```python
from build123d import *

# Parameters (mm, degrees)
F0_R           = 136.525
F1_DEPTH       = 3.175
F3_D           = 4.9784
F3_CSINK_D     = 9.8298
F3_CSINK_ANGLE = 82


with BuildPart() as f1:
    # F0 (on Top) → F1 (new body)
    with BuildSketch(Plane.XY):
        Circle(F0_R)
    extrude(amount=-F1_DEPTH)

    # F3 (through all)
    with Locations(Plane.XY):
        with Locations((-114.3, 0), (-57.15, 98.986704), (57.15, 98.986704), (114.3, 0), (57.15, -98.986704), (-57.15, -98.986704)):
            CounterSinkHole(F3_D / 2, F3_CSINK_D / 2, counter_sink_angle=F3_CSINK_ANGLE)


solid = f1.part
```
Read the model definition and answer for the solid it produces. Units are mm, in the model's axes. Coordinates: 2 decimals unless noted, no trailing zeros. Order: outer loops, then holes, each group sorted by start corner. A loop starts at its lowest first (then second) coordinate and runs counter-clockwise, first axis right, second up. Notation, with made-up numbers: (34, -17) - (75, -17) arc R20 ccw to (75, -11) - close; hole circle Ø3 at (15, 3.25). An arc over 180 degrees is marked (long way). Answer as a JSON object with one key per item and string values. Group by question number.
Item 1: Flat-ended cylindrical pins translate along their axes: P1, Ø10, axis at x = 79.5, y = 34, coming from the +Z side; P2, Ø8, axis at x = 57.15, y = 98.99, coming from the +Z side. Find the tip coordinate at first contact, or state that the pin passes through.
Item 2: Consider probe 1 along Y at (x, z) = (57.15, -2.95); probe 2 along X at (y, z) = (1, -2.8); probe 3 along X at (y, z) = (-99, -0.6). Determine where each line is inside the solid, lowest interval first. Write a range as from..to.
Item 3: Section A-A (z = -1.1) is taken. Give the vertices of the cut face in (x, y) (3 decimals), plus the area to 3 significant figures.
Item 4: The mould has two halves that part along X. Classify faces 1 (the face through (-136.393, 6.003, -1.565)), 2 (the face through (-116.71, -1, -2.65)), 3 (the face through (-2, 2, 0)): +X half, -X half, draft (parallel to the pull), parting line (faces both ways), or undercut.
Item 5: Section B-B (x = 99) is taken. Give the vertices of the cut face in (y, z) (3 decimals), plus the area to 3 significant figures.
Item 6: Section C-C (y = -80.5) is taken. Give the vertices of the cut face in (x, z) (3 decimals), plus the area to 3 significant figures.
Results are:
{
 "1": {"P1": "stops at z = 0", "P2": "stops at z = -1.05"},
 "2": {"probe 1": "y = -123.99..-101.48, -96.5..96.5, 101.48..123.99", "probe 2": "x = -136.52..-116.58, -112.02..112.02, 116.58..136.52", "probe 3": "x = -94.01..-61.54, -52.76..52.76, 61.54..94.01"},
 "3": {"outline": "circle Ø273.05 at (0, 0); hole circle Ø7.917 at (-114.3, 0); hole circle Ø7.917 at (-57.15, -98.987); hole circle Ø7.917 at (-57.15, 98.987); hole circle Ø7.917 at (57.15, -98.987); hole circle Ø7.917 at (57.15, 98.987); hole circle Ø7.917 at (114.3, 0)", "area": "58,300 mm^2"},
 "4": {"face 1": "parting line", "face 2": "undercut", "face 3": "draft"},
 "5": {"outline": "(-94.011, -3.175) - (94.011, -3.175) - (94.011, 0) - (-94.011, 0) - close", "area": "597 mm^2"},
 "6": {"outline": "(-110.267, -3.175) - (110.267, -3.175) - (110.267, 0) - (-110.267, 0) - close", "area": "700 mm^2"}
}
